For this review, take the finished solid that the model builds, in its own axes (mm). Face numbers are marked on the shaded views. A direction names the side the tool comes from. Coordinates: 2 decimals unless noted, no trailing zeros. Loops run counter-clockwise (first coordinate to the right, second up) from the corner with the lowest first, then second, coordinate; pieces in that order, holes last. Notation, with made-up numbers: M -11.75,66 L 14.25,66 A24 cw 14.25,94 Z; hole C 85,66.5 d10. An arc over 180 degrees is marked long. Put each result on its own line as item: value.
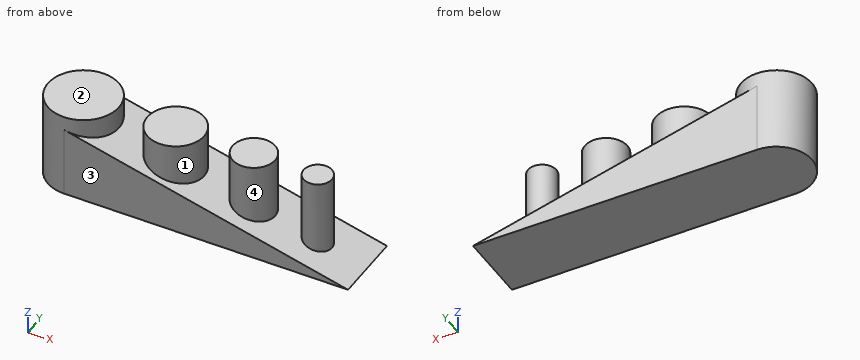
```python
from build123d import *

# Parameters (mm, degrees)
F0_W     = 40
F0_H     = 10
F1_DEPTH = 10
F3_DEPTH = 25
F4_R     = 5
F4_R_2   = 2
F4_R_3   = 4
F4_R_4   = 3
F5_DEPTH = 12


with BuildPart() as f1:
    # F0 (on Top) → F1 (new body)
    with BuildSketch(Plane.XY):
        with Locations((20, -5)):
            Rectangle(F0_W, F0_H)
    extrude(amount=F1_DEPTH)

    # F2 (on face) → F3 (cut)
    with BuildSketch(Plane.XZ.offset(10)):
        Polygon((40, 10), (0, 10), (40, 0), align=None)
    extrude(amount=-F3_DEPTH, mode=Mode.SUBTRACT)

    # F4 (on face) → F5 (join)
    with BuildSketch(Plane(origin=(0, 0, 0), x_dir=(1, 0, 0), z_dir=(0, 0, -1))):
        with Locations((0, 5)):
            Circle(F4_R)
        with Locations((33, 5)):
            Circle(F4_R_2)
        with Locations((13, 5)):
            Circle(F4_R_3)
        with Locations((24, 5)):
            Circle(F4_R_4)
    extrude(amount=-F5_DEPTH)


solid = f1.part
```
(1) Add section D-D (x = 24). Write out the cut boundary in (y, z).
Determined:
outline: M -10,0 L 0,0 L 0,4 L -2,4 L -2,12 L -8,12 L -8,4 L -10,4 Z
(2) Add section C-C (z = 7). Write out the cut boundary in (x, y).
Determined:
outline: M 0,-10 L 12,-10 L 12,-8.87 A4 ccw long 12,-1.13 L 12,0 L 0,0 A5 ccw Z; C 24,-5 d6; C 33,-5 d4
(3) For pin 1 (3 mm diameter, centred on y = -4, z = 8, fed in from +X); pin 2 (3 mm diameter, centred on x = 26.5, z = 9.5, fed in from -Y); pin 3 (3 mm diameter, centred on x = 13, z = 10.5, fed in from +Y), all flat-tipped, find the tip position at first contact; note any pin that passes through.
Determined:
pin 1: stops at x = 35
pin 2: stops at y = -7.83
pin 3: stops at y = -1
(4) Wall thickness on line 1 along X through (y, z) = (-4.75, 10.25); line 2 along X through (y, z) = (-6.5, 9); line 3 along X through (y, z) = (-4, 7): over which ranges is each line inside the solid? List them lowest first. Write a range as [from, to].
Determined:
line 1: x = [-4.99, 4.99], [9.01, 16.99], [21.01, 26.99], [31.02, 34.98]
line 2: x = [-4.77, 4.77], [9.29, 16.71], [21.4, 26.6], [31.68, 34.32]
line 3: x = [-4.9, 16.87], [21.17, 26.83], [31.27, 34.73]
(5) Add section A-A (y = -5). Write out the cut boundary in (x, z).
Determined:
outline: M -5,0 L 40,0 L 35,1.25 L 35,12 L 31,12 L 31,2.25 L 27,3.25 L 27,12 L 21,12 L 21,4.75 L 17,5.75 L 17,12 L 9,12 L 9,7.75 L 5,8.75 L 5,12 L -5,12 Z
(6) Tool access review of the marked faces 3 and 4: name each direction out of +Z, -Z, +X, -X, +Y, -Y from which nothing blocks a thin tool from reaching the whole face with its end or side.
Determined:
face 3: +Z, -Z, +X, -X, -Y
face 4: +Z
(7) Add section B-B (x = 4). Write out the cut boundary in (y, z), plus the area to 3 significant figures.
Determined:
outline: M -10,0 L 0,0 L 0,9 L -2,9 L -2,12 L -8,12 L -8,9 L -10,9 Z
area: 108 mm^2
(8) Draft analysis for pull direction X (two halves, no side actions). For the marked faces 1 and 2, state which applies: +X half, -X half, draft (parallel to the pull), parting line (faces both ways), or undercut.
Determined:
face 1: undercut
face 2: draft
